Build history of the part. All positions in model axes, mm. A direction names the side the tool comes from. Give positions to 0.01 mm unless a question says otherwise; leave off trailing zeros. Write each loop counter-clockwise with the first axis right and the second up, starting at its lowest first coordinate (ties: lowest second). Pieces come first, ordered by that corner, then holes. Notation, with made-up numbers: M 5,79 L 17,79 A24 ccw 17,92 Z; hole C 50.5,28.25 d1. An arc over 180 degrees is marked long. Return JSON: item names as keys, results as strings. Group by question number.
Q1. Pull direction Z, two halves, no side cores. Call faces 5 (the flat face through (3, -4, 0)), 6 (the flat face through (-2.339, -4, 14)), 7 (the flat face through (5, -0.489, 10)): +Z half, -Z half, draft (parallel to the pull), parting line (faces both ways), or undercut.
Q2. Band-saw the part on A-A, the plane z = 10. Give the cut face in (x, y).
Q3. Band-saw the part on B-B, the plane z = 5. Give the cut face in (x, y), then the cut area to 3 significant figures.
Q4. Flat gauge pins, fed straight in: pin 1 Ø2.5 at (x, z) = (18.66, 10) entering from -Y; pin 2 Ø0.5 at (y, z) = (-2, 7.5) entering from +X; pin 3 Ø3 at (y, z) = (-8, 10.5) entering from +X. Where does each tip first touch, or does it go through?
Q5. Tool access for faces 1 (the cylindrical face through (19.091, -4.468, 14.325)), 2 (the flat face through (13.661, -7, 10)), 3 (the flat face through (18, -1.489, 10)), 4 (the cylindrical face through (-5.04, -4.45, 1.53)): list every direction of +Z, -Z, +X, -X, +Y, -Y with a clear straight run to the whole face (end or side of a thin tool).
Q6. Wall check: probe 1 along Y at (x, z) = (18, 3.5); probe 2 along X at (y, z) = (-3.85, 10); probe 3 along Z at (x, y) = (-2.5, -2). Give the ranges that are in metal, low to high.
from build123d import *

# Parameters (mm, degrees)
SKETCH1_R                  = 3
SKETCH1_R_2                = 2
BOSS_EXTRUDE1_DEPTH        = 20
SKETCH2_R                  = 3
CUT_EXTRUDE1_DEPTH         = 7
M2X0_4_TAPPED_HOLE1_REACH  = 31.847
M2X0_4_TAPPED_HOLE1_BORE_R = 0.8
M2X0_4_TAPPED_HOLE2_REACH  = 31.982
M2X0_4_TAPPED_HOLE2_BORE_R = 0.8
M2X0_4_TAPPED_HOLE3_D      = 1.6
M2X0_4_TAPPED_HOLE3_DEPTH  = 3


with BuildPart() as part:
    # Sketch1 → Boss-Extrude1 (new body)
    with BuildSketch(Plane.XY):
        Polygon((20.660587733, -2.988994126), (20.660587733, -5.988994126), (13.660587733, -5.988994126), (13.660587733, -8.488994126), (-9.339412267, -8.488994126), (-9.339412267, -2.742720205), (-9.339412267, -0.488994126), (20.660587733, -0.488994126), (20.660587733, -1.488994126), (15.660587733, -1.488994126), (15.660587733, -2.988994126), align=None)
        with Locations((6.188452756, -4.06657859)):
            Circle(SKETCH1_R, mode=Mode.SUBTRACT)
        with Locations((12.160587733, -3.488994126)):
            Circle(SKETCH1_R_2, mode=Mode.SUBTRACT)
    extrude(amount=BOSS_EXTRUDE1_DEPTH)

    # Sketch2 → Cut-Extrude1 (cut)
    with BuildSketch(Plane.ZY.offset(9.339412267)):
        with Locations(Location((6, -4.488994126, 0), (0, 0, 270))):
            Circle(SKETCH2_R)
        with Locations(Location((14, -4.488994126, 0), (0, 0, 270))):
            Circle(SKETCH2_R)
    extrude(amount=-CUT_EXTRUDE1_DEPTH, mode=Mode.SUBTRACT)

    # M2x0.4 Tapped Hole1 bore → M2x0.4 Tapped Hole1 (cut, up to next)
    with BuildSketch(Plane(origin=(0, -8.488994126, 0), x_dir=(-1, 0, 0), z_dir=(0, -1, 0)), mode=Mode.PRIVATE) as m2x0_4_tapped_hole1_sk1:
        with Locations((-12.160587733, -10)):
            Circle(M2X0_4_TAPPED_HOLE1_BORE_R)
    m2x0_4_tapped_hole1_tool1 = extrude(m2x0_4_tapped_hole1_sk1.sketch, amount=-M2X0_4_TAPPED_HOLE1_REACH, mode=Mode.PRIVATE) & part.part
    # M2x0.4 Tapped Hole1 bore → M2x0.4 Tapped Hole1 (cut, up to next)
    with BuildSketch(Plane(origin=(0, -8.488994126, 0), x_dir=(-1, 0, 0), z_dir=(0, -1, 0)), mode=Mode.PRIVATE) as m2x0_4_tapped_hole1_sk2:
        with Locations((-6.188452756, -10)):
            Circle(M2X0_4_TAPPED_HOLE1_BORE_R)
    m2x0_4_tapped_hole1_tool2 = extrude(m2x0_4_tapped_hole1_sk2.sketch, amount=-M2X0_4_TAPPED_HOLE1_REACH, mode=Mode.PRIVATE) & part.part
    add(m2x0_4_tapped_hole1_tool1.solids().sort_by_distance((12.160588, -8.488994, 10))[0], mode=Mode.SUBTRACT)
    add(m2x0_4_tapped_hole1_tool2.solids().sort_by_distance((6.188453, -8.488994, 10))[0], mode=Mode.SUBTRACT)

    # M2x0.4 Tapped Hole2 bore → M2x0.4 Tapped Hole2 (cut, up to next)
    with BuildSketch(Plane(origin=(0, 0, 0), x_dir=(-1, 0, 0), z_dir=(0, 0, -1)), mode=Mode.PRIVATE) as m2x0_4_tapped_hole2_sk1:
        with Locations((5.839412267, -4.488994126)):
            Circle(M2X0_4_TAPPED_HOLE2_BORE_R)
    m2x0_4_tapped_hole2_tool1 = extrude(m2x0_4_tapped_hole2_sk1.sketch, amount=-M2X0_4_TAPPED_HOLE2_REACH, mode=Mode.PRIVATE) & part.part
    m2x0_4_tapped_hole2 = m2x0_4_tapped_hole2_tool1.solids().sort_by_distance((-5.839412, -4.488994, 0))[0]
    add(m2x0_4_tapped_hole2, mode=Mode.SUBTRACT)

    # Mirror1: M2x0.4 Tapped Hole2 across plane
    add(m2x0_4_tapped_hole2.mirror(Plane(origin=(0, 0, 10), x_dir=(1, 0, 0), z_dir=(0, 0, -1))), mode=Mode.SUBTRACT)

    # M2x0.4 Tapped Hole3
    with Locations(Plane(origin=(0, -5.988994126, 0), x_dir=(-1, 0, 0), z_dir=(0, -1, 0))):
        with Locations((-18.660587733, -5), (-18.660587733, -15), (-18.660587733, -10)):
            Hole(M2X0_4_TAPPED_HOLE3_D / 2, depth=M2X0_4_TAPPED_HOLE3_DEPTH)


solid = part.part
From the geometry:
{
 "1": {"face 5": "-Z half", "face 6": "undercut", "face 7": "draft"},
 "2": {"outline": "M -9.34,-8.49 L 5.39,-8.49 L 5.39,-6.96 A3 cw long 6.99,-6.96 L 6.99,-8.49 L 11.36,-8.49 L 11.36,-5.32 A2 cw long 12.96,-5.32 L 12.96,-8.49 L 13.66,-8.49 L 13.66,-5.99 L 17.86,-5.99 L 17.86,-2.99 L 15.66,-2.99 L 15.66,-1.49 L 20.66,-1.49 L 20.66,-0.49 L -9.34,-0.49 Z; M 19.46,-5.99 L 20.66,-5.99 L 20.66,-2.99 L 19.46,-2.99 Z"},
 "3": {"outline": "M -9.34,-8.49 L 13.66,-8.49 L 13.66,-5.99 L 17.86,-5.99 L 17.86,-2.99 L 15.66,-2.99 L 15.66,-1.49 L 20.66,-1.49 L 20.66,-0.49 L -9.34,-0.49 L -9.34,-1.66 L -2.34,-1.66 L -2.34,-7.32 L -9.34,-7.32 Z; M 19.46,-5.99 L 20.66,-5.99 L 20.66,-2.99 L 19.46,-2.99 Z; hole C 6.19,-4.07 d6; hole C 12.16,-3.49 d4", "area": "130 mm^2"},
 "4": {"pin 1": "stops at y = -5.99", "pin 2": "stops at x = 15.66", "pin 3": "stops at x = 13.66"},
 "5": {"face 1": "-Y", "face 2": "+Z, -Z, +X, -Y", "face 3": "+Z, -Z, +X", "face 4": "-Z"},
 "6": {"probe 1": "y = -5.99 to -2.99, -1.49 to -0.49", "probe 2": "x = -9.34 to 3.2, 9.18 to 10.19, 14.13 to 17.86, 19.46 to 20.66", "probe 3": "z = 0 to 4.33, 7.67 to 12.33, 15.67 to 20"}
}
